```python
from build123d import *

# Parameters (mm, degrees)
SKETCH2_W                      = 30
SKETCH2_H                      = 17
BOSS_EXTRUDE1_DEPTH            = 50
CUT_EXTRUDE4_REACH             = 64.33
SKETCH7_R                      = 10.025
F_3_0MM_DOWEL_HOLE1_D          = 3.4
F_3_0MM_DOWEL_HOLE1_DEPTH      = 5.5
BOSS_EXTRUDE2_REACH            = 62.374
FILLET1_R                      = 1
CUT_EXTRUDE7_REACH             = 70.884
SKETCH13_W                     = 33.931840249
SKETCH13_H                     = 30
CUT_EXTRUDE7_DIRECTION_2_DEPTH = 10


with BuildPart() as part:
    # Sketch2 → Boss-Extrude1 (new body)
    with BuildSketch(Plane(origin=(0, 0, 0), x_dir=(0, 0, -1), z_dir=(1, 0, 0))):
        Polygon((19, -14), (3.999996995, -14), (0, -17.999996995), (-3.999996995, -14), (-19, -14), (-19, 14), (19, 14), align=None)
        Rectangle(SKETCH2_W, SKETCH2_H, mode=Mode.SUBTRACT)
    extrude(amount=BOSS_EXTRUDE1_DEPTH)

    # Sketch7 → Cut-Extrude4 (cut, up to next)
    with BuildSketch(Plane(origin=(0, 14, 0), x_dir=(1, 0, 0), z_dir=(0, 1, 0)), mode=Mode.PRIVATE) as cut_extrude4_sk1:
        with Locations(Location((25, 0, 0), (0, 0, 270))):
            Circle(SKETCH7_R)
    cut_extrude4_tool1 = extrude(cut_extrude4_sk1.sketch, amount=-CUT_EXTRUDE4_REACH, mode=Mode.PRIVATE) & part.part
    add(cut_extrude4_tool1.solids().sort_by_distance((25, 14, 0))[0], mode=Mode.SUBTRACT)

    # Ø3.0mm Dowel Hole1
    with Locations(Plane(origin=(0, 14, 0), x_dir=(1, 0, 0), z_dir=(0, 1, 0))):
        with Locations((18, -12.124355653), (18, 12.124355653), (39, 0)):
            Hole(F_3_0MM_DOWEL_HOLE1_D / 2, depth=F_3_0MM_DOWEL_HOLE1_DEPTH)

    # Boss-Extrude2: up to this face of the body (flat: up to its plane)
    boss_extrude2_end = Plane(part.part.faces().sort_by_distance((25, 14, 18.371987261))[0])
    # Sketch6 → Boss-Extrude2 (add, up to the picked face)
    with BuildSketch(Plane(origin=(0, -14, 0), x_dir=(1, 0, 0), z_dir=(0, 1, 0)), mode=Mode.PRIVATE) as boss_extrude2_sk1:
        with BuildLine():
            Line((60, 3.6), (59.5, 3.6))
            Line((59.5, 3.6), (59.5, 3.1))
            Line((59.5, 3.1), (58.2, 3.1))
            Line((58.2, 3.1), (58.2, 5.5))
            Line((58.2, 5.5), (56.560660172, 5.5))
            Line((56.560660172, 5.5), (54.485786438, 3.425126266))
            ThreePointArc((54.485786438, 3.425126266), (54.052240935, 2.776279568), (53.9, 2.010912703))
            Line((53.9, 2.010912703), (53.9, -2.010912703))
            ThreePointArc((53.9, -2.010912703), (54.052240935, -2.776279568), (54.485786438, -3.425126266))
            Line((54.485786438, -3.425126266), (56.560660172, -5.5))
            Line((56.560660172, -5.5), (58.2, -5.5))
            Line((58.2, -5.5), (58.2, -3.1))
            Line((58.2, -3.1), (59.5, -3.1))
            Line((59.5, -3.1), (59.5, -3.6))
            Line((59.5, -3.6), (60, -3.6))
            Line((60, -3.6), (60, -10))
            Line((60, -10), (50, -10))
            Line((50, -10), (50, 10))
            Line((50, 10), (60, 10))
            Line((60, 10), (60, 3.6))
        make_face()
    boss_extrude2_tool1 = split(extrude(boss_extrude2_sk1.sketch, amount=BOSS_EXTRUDE2_REACH, mode=Mode.PRIVATE), bisect_by=boss_extrude2_end, keep=Keep.BOTH, mode=Mode.PRIVATE)
    add(boss_extrude2_tool1.solids().sort_by(Axis((59.75, -14, -3.823607), (0, 1, 0)))[0])

    # Fillet1
    fillet1_edges = [part.edges().sort_by_distance(p)[0] for p in [
        (55, 14, -10),
        (0, -8.5, 0),
        (0, 0, 15),
        (0, 8.5, 0),
        (0, 0, -15),
        (0, -14, 11.499998498),
        (0, -15.999998498, 1.999998498),
        (0, -15.999998498, -1.999998498),
        (0, -14, -11.499998498),
        (0, 14, 0),
        (25, -14, -19),
        (50, 0, -19),
        (25, 14, -19),
        (0, 0, -19),
        (25, 14, 19),
        (50, 0, 19),
        (25, -14, 19),
        (0, 0, 19),
        (50, 14, -14.5),
        (50, 11.25, -10),
        (55, 14, 10),
        (50, 14, 14.5),
        (60, 0, -10),
        (60, 0, 10),
        (60, -14, 6.8),
        (60, -14, -6.8),
        (60, 14, 6.8),
        (60, 14, -6.8),
    ]]
    fillet(fillet1_edges, radius=FILLET1_R)

    # Sketch13 → Cut-Extrude7 (cut, up to next)
    with BuildSketch(Plane.XZ.offset(14), mode=Mode.PRIVATE) as cut_extrude7_sk1:
        with Locations((27.606274686, 0)):
            Rectangle(SKETCH13_W, SKETCH13_H)
    cut_extrude7_tool1 = extrude(cut_extrude7_sk1.sketch, amount=-CUT_EXTRUDE7_REACH, mode=Mode.PRIVATE) & part.part
    add(cut_extrude7_tool1.solids().sort_by_distance((27.606275, -14, 0))[0], mode=Mode.SUBTRACT)

    # Sketch13 → Cut-Extrude7 direction 2 (cut)
    with BuildSketch(Plane.XZ.offset(14)):
        with Locations((27.606274686, 0)):
            Rectangle(SKETCH13_W, SKETCH13_H)
    extrude(amount=CUT_EXTRUDE7_DIRECTION_2_DEPTH, mode=Mode.SUBTRACT)


solid = part.part
```
Geometry check sheet. Reference: the model listing, model coordinates, mm. A direction names the side the tool comes from. Give positions to 0.01 mm unless a question says otherwise; leave off trailing zeros. Order: outer loops, then holes, each group sorted by start corner. A loop starts at its lowest first (then second) coordinate and runs counter-clockwise, first axis right, second up.
1. Access from +Z, -Z, +X, -X, +Y, -Y to the whole of each face (thin tool, end or side, straight path). Record for faces 1 (the face through (60, 0, -6)), 2 (the face through (53.9, 0, 0)), 3 (the face through (0.285, -15.671, -1.904)), 4 (the face through (58.2, 0, -4)), 5 (the face through (25.6, 8.5, 10.2)).
2. Gauge pin test, flat ends, axial feed: pin 1 Ø1.9 at (y, z) = (-1, -4) entering from -X; pin 2 Ø6 at (y, z) = (-6, -13.5) entering from +X; pin 3 Ø5 at (x, z) = (32.5, 8) entering from -Y. Record the tip position at first contact, or that the pin passes through.
3. Thickness scan on L1, parallel to Z at x = 39.5, y = 7; L2, parallel to Y at x = 9, z = -9; L3, parallel to Z at x = 18, y = 9. Record the ranges inside material, lowest first.
4. Section check A-A, the plane x = 25. Enter the section's corners in (y, z) (3 decimals), and give its area (3 significant figures).
5. Section check B-B, the plane z = 7.5. Enter the section's corners in (x, y), and give its area (3 significant figures).
6. Section check D-D, the plane x = 18. Enter the section's corners in (y, z).
7. Section check C-C, the plane x = 5.5. Enter the section's corners in (y, z).
8. Release check for a two-part mould opening along Z. For faces 6 (the face through (25, 0, -19)), 7 (the face through (55.51, -0.2, 4.45)), 8 (the face through (0, -10, -1)) record: pulls with the +Z half, pulls with the -Z half, needs draft (parallel to the pull), parting line crosses it, or undercut.
Values follow:
1. face 1: +Z, -Z, +X, +Y, -Y
1. face 2: +X, +Y, -Y
1. face 3: -Z, -X, -Y
1. face 4: +Y, -Y
1. face 5: -X
2. pin 1: stops at x = 50
2. pin 2: stops at x = 50
2. pin 3: stops at y = 8.5
3. L1: z = -19 to -15, 15 to 19
3. L2: y = -14 to -8.5, 8.5 to 14
3. L3: z = -19 to -13.82, -10.42 to -7.18, 7.18 to 10.42, 13.82 to 19
4. outline: (-14, -18) arc R1 ccw to (-13, -19) - (13, -19) arc R1 ccw to (14, -18) - (14, -10.025) - (8.5, -10.025) - (8.5, -15) - (-14, -15) - close; (-14, 15) - (8.5, 15) - (8.5, 10.025) - (14, 10.025) - (14, 18) arc R1 ccw to (13, 19) - (-13, 19) arc R1 ccw to (-14, 18) - close
4. area: 278 mm2
5. outline: (0, -13) arc R1 ccw to (1, -14) - (10.64, -14) - (10.64, -8.5) - (1, -8.5) arc R1 ccw to (0, -9.5) - close; (0, 9.5) arc R1 ccw to (1, 8.5) - (18.35, 8.5) - (18.35, 14) - (1, 14) arc R1 ccw to (0, 13) - close; (31.65, 8.5) - (50, 8.5) - (50, -8.5) - (44.57, -8.5) - (44.57, -14) - (59, -14) arc R1 ccw to (60, -13) - (60, 13) arc R1 ccw to (59, 14) - (31.65, 14) - close
5. area: 569 mm2
6. outline: (-14, -18) arc R1 ccw to (-13, -19) - (13, -19) arc R1 ccw to (14, -18) - (14, -13.82) - (8.5, -13.82) - (8.5, -15) - (-14, -15) - close; (-14, 15) - (8.5, 15) - (8.5, 13.82) - (14, 13.82) - (14, 18) arc R1 ccw to (13, 19) - (-13, 19) arc R1 ccw to (-14, 18) - close; (8.5, -10.42) - (14, -10.42) - (14, -7.18) - (8.5, -7.18) - close; (8.5, 7.18) - (14, 7.18) - (14, 10.42) - (8.5, 10.42) - close
7. outline: (-18, 0) - (-14, -4) - (-14, -18) arc R1 ccw to (-13, -19) - (13, -19) arc R1 ccw to (14, -18) - (14, 18) arc R1 ccw to (13, 19) - (-13, 19) arc R1 ccw to (-14, 18) - (-14, 4) - close; hole (-8.5, -15) - (8.5, -15) - (8.5, 15) - (-8.5, 15) - close
8. face 6: pulls with the -Z half
8. face 7: undercut
8. face 8: needs draft
